from build123d import *

# Parameters (mm, degrees)
SKETCH1_W           = 3
SKETCH1_H           = 38.7
SKETCH1_H_2         = 3
SKETCH1_W_2         = 6
SKETCH1_H_3         = 3.5
BOSS_EXTRUDE1_DEPTH = 11
SKETCH2_R           = 1.5
CUT_EXTRUDE1_DEPTH  = 10
SKETCH3_R           = 1.5
CUT_EXTRUDE2_DEPTH  = 10
FILLET1_R           = 2


with BuildPart() as part:
    # Sketch1 → Boss-Extrude1 (new, symmetric)
    with BuildSketch(Plane(origin=(0, 0, 0), x_dir=(0, 0, -1), z_dir=(1, 0, 0))):
        with Locations((0, -1.5)):
            Rectangle(SKETCH1_W, SKETCH1_H)
        with Locations((0, 19.35)):
            Rectangle(SKETCH1_W, SKETCH1_H_2)
        Polygon((23.05, 20.85), (1.5, 20.85), (1.5, 17.85), (17.035825545, 17.85), (17.05, 17.85), (23.05, 17.85), align=None)
        with Locations((20.05, 16.1)):
            Rectangle(SKETCH1_W_2, SKETCH1_H_3)
    extrude(amount=BOSS_EXTRUDE1_DEPTH, both=True)

    # Sketch2 → Cut-Extrude1 (cut)
    with BuildSketch(Plane.XY.offset(1.5)):
        with Locations((0, -14.85)):
            Circle(SKETCH2_R)
    extrude(amount=-CUT_EXTRUDE1_DEPTH, mode=Mode.SUBTRACT)

    # Sketch3 → Cut-Extrude2 (cut)
    with BuildSketch(Plane(origin=(0, 20.85, 0), x_dir=(1, 0, 0), z_dir=(0, 1, 0))):
        with Locations(Location((-8, 20.05, 0), (0, 0, 270))):
            Circle(SKETCH3_R)
        with Locations(Location((8, 20.05, 0), (0, 0, 90))):
            Circle(SKETCH3_R)
    extrude(amount=-CUT_EXTRUDE2_DEPTH, mode=Mode.SUBTRACT)

    # Fillet1
    # the kernel refuses this fillet: 2 mm, written as the material it adds along each edge
    with BuildSketch(Plane(origin=(-11, 17.85, -17.05), x_dir=(0, 0, 1), z_dir=(1, 0, 0)), Plane(origin=(-11, 17.85, -1.5), x_dir=(0, -1, 0), z_dir=(1, 0, 0))) as fillet1_piece_1:
        with BuildLine():
            CenterArc((FILLET1_R, FILLET1_R), FILLET1_R, 180, 90)
            Line((0, FILLET1_R), (0, 0))
            Line((0, 0), (FILLET1_R, 0))
        make_face()
    extrude(amount=22)
    # the kernel refuses this fillet: 2 mm, written as the material it takes off along each edge
    with BuildSketch(Plane(origin=(-9, 18.85, -0.5), x_dir=(-1, 0, 0), z_dir=(0, 0, 1))) as fillet1_2_piece_1_section:
        Polygon((0, 0), (FILLET1_R, 0), (FILLET1_R, -FILLET1_R), (0, -FILLET1_R), align=None)
    fillet1_2_piece_1 = extrude(amount=FILLET1_R, mode=Mode.PRIVATE)
    fillet1_2_piece_1 = fillet1_2_piece_1 - Plane(origin=(-9, 18.85, -0.5), x_dir=(0.7071067811865475, -0.7071067811865475, 0), z_dir=(0, 0, 1)) * Sphere(FILLET1_R, mode=Mode.PRIVATE)
    add(fillet1_2_piece_1, mode=Mode.SUBTRACT)
    with BuildSketch(Plane(origin=(-11, 18.85, 1.5), x_dir=(1, 0, 0), z_dir=(0, -1, 0))) as fillet1_2_piece_2:
        with BuildLine():
            CenterArc((FILLET1_R, -FILLET1_R), FILLET1_R, 90, 90)
            Line((0, -FILLET1_R), (0, 0))
            Line((0, 0), (FILLET1_R, 0))
        make_face()
    extrude(amount=44.7, mode=Mode.SUBTRACT)
    with BuildSketch(Plane(origin=(-11, 20.85, -28.05), x_dir=(0, -1, 0), z_dir=(0, 0, 1))) as fillet1_2_piece_3:
        with BuildLine():
            CenterArc((FILLET1_R, FILLET1_R), FILLET1_R, 180, 90)
            Line((0, FILLET1_R), (0, 0))
            Line((0, 0), (FILLET1_R, 0))
        make_face()
    extrude(amount=27.55, mode=Mode.SUBTRACT)
    with BuildSketch(Plane(origin=(16, 20.85, 1.5), x_dir=(0, -1, 0), z_dir=(-1, 0, 0))) as fillet1_2_piece_4:
        with BuildLine():
            CenterArc((FILLET1_R, -FILLET1_R), FILLET1_R, 90, 90)
            Line((0, -FILLET1_R), (0, 0))
            Line((0, 0), (FILLET1_R, 0))
        make_face()
    extrude(amount=25, mode=Mode.SUBTRACT)
    with BuildSketch(Plane(origin=(16, 20.85, -23.05), x_dir=(0, 0, 1), z_dir=(-1, 0, 0))) as fillet1_2_piece_5:
        with BuildLine():
            CenterArc((FILLET1_R, -FILLET1_R), FILLET1_R, 90, 90)
            Line((0, -FILLET1_R), (0, 0))
            Line((0, 0), (FILLET1_R, 0))
        make_face()
    extrude(amount=32, mode=Mode.SUBTRACT)


solid = part.part
Verification items for the finished model (mm, model axes). A direction names the side the tool comes from. Round coordinates to 2 decimals unless told otherwise and drop trailing zeros. Order: outer loops, then holes, each group sorted by start corner. A loop starts at its lowest first (then second) coordinate and runs counter-clockwise, first axis right, second up.
1. Section check B-B on y = -14.85. Record the cut outline in (x, z).
Final values:
outline: (-11, -1.5) - (-1.5, -1.5) - (-1.5, 1.5) - (-9, 1.5) arc R2 ccw to (-11, -0.5) - close; (1.5, -1.5) - (11, -1.5) - (11, 1.5) - (1.5, 1.5) - close
2. Section check A-A on x = 0. Record the cut outline in (y, z), then the cut area to 3 significant figures.
Final values:
outline: (-20.85, -1.5) - (-16.35, -1.5) - (-16.35, 1.5) - (-20.85, 1.5) - close; (-13.35, -1.5) - (15.85, -1.5) arc R2 cw to (17.85, -3.5) - (17.85, -15.05) arc R2 cw to (15.85, -17.05) - (14.35, -17.05) - (14.35, -23.05) - (18.85, -23.05) arc R2 ccw to (20.85, -21.05) - (20.85, -0.5) arc R2 ccw to (18.85, 1.5) - (-13.35, 1.5) - close
area: 202 mm2
3. Release check for a two-part mould opening along X. For faces 1 (the cylindrical face through (9.464, 17.646, -19.725)), 2 (the cylindrical face through (-0.15, 17.28, -2.1)), 3 (the cylindrical face through (-10.4, 20.28, -11.93)) record: +X half, -X half, draft (parallel to the pull), parting line (faces both ways), or undercut.
Final values:
face 1: undercut
face 2: draft
face 3: -X half
4. Section check C-C on z = -20.05. Record the cut outline in (x, y), then the cut area to 3 significant figures.
Final values:
outline: (-11, 14.35) - (-9.5, 14.35) - (-9.5, 20.79) arc R2 ccw to (-11, 18.85) - close; (-6.5, 14.35) - (6.5, 14.35) - (6.5, 20.85) - (-6.5, 20.85) - close; (9.5, 14.35) - (11, 14.35) - (11, 20.85) - (9.5, 20.85) - close
area: 103 mm2
5. Thickness scan on L1, parallel to X at y = 17, z = -20.05; L2, parallel to Y at x = -2, z = -17.25; L3, parallel to Y at x = -5.5, z = -5.75. Record the ranges inside material, lowest first.
Final values:
L1: x = -11 to -9.5, -6.5 to 6.5, 9.5 to 11
L2: y = 14.35 to 20.85
L3: y = 17.85 to 20.85
6. Go/stop test with flat-tipped pins: P1, Ø6, axis at x = -4, y = -13.5, coming from the -Z side; P2, Ø12.5, axis at x = -4, z = -6.5, coming from the -Y side; P3, Ø5, axis at x = -8, z = -20.05, coming from the -Y side; P4, Ø4, axis at x = 0.5, z = -6, coming from the -Y side. Record where each tip stops, or that it passes through.
Final values:
P1: stops at z = -1.5
P2: stops at y = -20.85
P3: stops at y = 14.35
P4: stops at y = 17.85
7. Access from +Z, -Z, +X, -X, +Y, -Y to the whole of each face (thin tool, end or side, straight path). Record for faces 4 (the cylindrical face through (1.14, 20.25, 0.93)), 5 (the flat face through (0, 15, -17.05)), 6 (the flat face through (0, 14.35, -20)).
Final values:
face 4: +Z, +X, -X, +Y
face 5: +X, -X, -Y
face 6: -Z, +X, -X, -Y
8. Section check D-D on x = -6. Record the cut outline in (y, z).
Final values:
outline: (-20.85, -1.5) - (15.85, -1.5) arc R2 cw to (17.85, -3.5) - (17.85, -15.05) arc R2 cw to (15.85, -17.05) - (14.35, -17.05) - (14.35, -23.05) - (18.85, -23.05) arc R2 ccw to (20.85, -21.05) - (20.85, -0.5) arc R2 ccw to (18.85, 1.5) - (-20.85, 1.5) - close
